Part model, mm, in its own coordinate system. Face numbers are marked on the shaded views. A direction names the side the tool comes from. Coordinates: 2 decimals unless noted, no trailing zeros. Write each loop counter-clockwise with the first axis right and the second up, starting at its lowest first coordinate (ties: lowest second). Pieces come first, ordered by that corner, then holes. Notation, with made-up numbers: (74.25, -32) -> (98.25, -32) arc R18 ccw to (98.25, -27) -> close; hole circle Ø11 at (20, -3.5). An arc over 180 degrees is marked (long way). One line per question, with ' | ' between items. Start each with the question number.
Item 1: Saw through at A-A (y = 0). List the corners of the cut face in (x, z), and give its area (3 significant figures).
Item 2: Pin check, flat tips, straight feed: pin 1 (1.7 mm diameter, centred on y = -2.5, z = 2, fed in from +X); pin 2 (4 mm diameter, centred on y = 1, z = -1, fed in from -X); pin 3 (10 mm diameter, centred on x = -6, y = 3, fed in from +Z); pin 4 (6 mm diameter, centred on x = 5.5, y = -5.5, fed in from -Z). Stop position of each tip, or through.
Item 3: Two-plate mould, pull along Y, no slides. Class the marked faces 1, 2 and 3: pulls with the +Y half, pulls with the -Y half, needs draft (parallel to the pull), parting line crosses it, or undercut.
Item 4: Saw through at B-B (x = -5.5). Count the separate pieces of the cut face and the enclosed holes in it, and give its area (4 significant figures).
Item 5: Probe probe 1 along X at (y, z) = (-3, 3.75); probe 2 along X at (y, z) = (1, -0.75); probe 3 along Y at (x, z) = (-1, 3.5). List the from-to ranges inside material, lowest first. Write a range as [from, to].
Item 6: 3-axis set-ups, long thin cutter, end or side, ignore diameter. For the marked faces 4, 5 and 6: which of +Z, -Z, +X, -X, +Y, -Y reach the whole face in a straight line?
from build123d import *

# Parameters (mm, degrees)
IZIM1_R                          = 14.3
Y_KSEKLIK_EKSTR_ZYON2_DEPTH      = 3
IZIM2_R                          = 13
Y_KSEKLIK_EKSTR_ZYON3_DEPTH      = 1.5
IZIM3_R                          = 13
Y_KSEKLIK_EKSTR_ZYON4_DEPTH      = 1.5
KES_EKSTR_ZYON1_DEPTH            = 7
KES_EKSTR_ZYON3_DEPTH            = 7
IZIM6_R                          = 16
IZIM6_R_2                        = 13
Y_KSEKLIK_EKSTR_ZYON5_DEPTH      = 0.35
Y_KSEKLIK_EKSTR_ZYON5_DEPTH_BACK = 6.65
RADYUS1_R                        = 1
RADYUS2_R                        = 1


with BuildPart() as part:
    # Çizim1 → Yükseklik-Ekstrüzyon2 (new body)
    with BuildSketch(Plane.XY):
        Circle(IZIM1_R)
    extrude(amount=Y_KSEKLIK_EKSTR_ZYON2_DEPTH)

    # Çizim2 → Yükseklik-Ekstrüzyon3 (add)
    with BuildSketch(Plane.XY.offset(3)):
        Circle(IZIM2_R)
    extrude(amount=Y_KSEKLIK_EKSTR_ZYON3_DEPTH)

    # Çizim3 → Yükseklik-Ekstrüzyon4 (add)
    with BuildSketch(Plane(origin=(0, 0, 0), x_dir=(-1, 0, 0), z_dir=(0, 0, -1))):
        Circle(IZIM3_R)
    extrude(amount=Y_KSEKLIK_EKSTR_ZYON4_DEPTH)

    # Çizim4 → Kes-Ekstrüzyon1 (cut)
    with BuildSketch(Plane.XY.offset(4.5)):
        with BuildLine():
            add(Edge.make_bspline(
                [(-0.547346557, 3.558147235), (0.233958313, 12.343828963), (-3.6, 11.184922888)],
                knots=[0, 0, 0, 0.973142828, 0.973142828, 0.973142828], degree=2))
            ThreePointArc((-3.6, 11.184922888), (-3.707741279, 11.149670605), (-3.81513744, 11.113380508))
            ThreePointArc((-3.81513744, 11.113380508), (-10.175798494, 5.875), (-11.532038562, -2.252684312))
            ThreePointArc((-11.532038562, -2.252684312), (-11.509768628, -2.363837165), (-11.48642736, -2.47476999))
            add(Edge.make_bspline(
                [(-3.355119175, -1.305057594), (-10.573090305, -6.374528324), (-11.48642736, -2.47476999)],
                knots=[0, 0, 0, 0.973142828, 0.973142828, 0.973142828], degree=2))
            ThreePointArc((-3.355119175, -1.305057594), (-3.117691454, 1.8), (-0.547346557, 3.558147235))
        make_face()
        with BuildLine():
            add(Edge.make_bspline(
                [(3.355119175, -1.305057594), (10.573090305, -6.374528324), (11.48642736, -2.47476999)],
                knots=[0, 0, 0, 0.973142828, 0.973142828, 0.973142828], degree=2))
            ThreePointArc((11.48642736, -2.47476999), (11.509768628, -2.363837165), (11.532038562, -2.252684312))
            ThreePointArc((11.532038562, -2.252684312), (10.175798494, 5.875), (3.81513744, 11.113380508))
            ThreePointArc((3.81513744, 11.113380508), (3.707741279, 11.149670605), (3.6, 11.184922888))
            add(Edge.make_bspline(
                [(0.547346557, 3.558147235), (-0.233958313, 12.343828963), (3.6, 11.184922888)],
                knots=[0, 0, 0, 0.973142828, 0.973142828, 0.973142828], degree=2))
            ThreePointArc((0.547346557, 3.558147235), (3.117691454, 1.8), (3.355119175, -1.305057594))
        make_face()
        with BuildLine():
            add(Edge.make_bspline(
                [(-2.807772617, -2.253089641), (-10.807048618, -5.969300639), (-7.88642736, -8.710152897)],
                knots=[0, 0, 0, 0.973142828, 0.973142828, 0.973142828], degree=2))
            ThreePointArc((-7.88642736, -8.710152897), (-7.802027349, -8.785833441), (-7.716901122, -8.860696196))
            ThreePointArc((-7.716901122, -8.860696196), (0, -11.75), (7.716901122, -8.860696196))
            ThreePointArc((7.716901122, -8.860696196), (7.802027349, -8.785833441), (7.88642736, -8.710152897))
            add(Edge.make_bspline(
                [(2.807772617, -2.253089641), (10.807048618, -5.969300639), (7.88642736, -8.710152897)],
                knots=[0, 0, 0, 0.973142828, 0.973142828, 0.973142828], degree=2))
            ThreePointArc((2.807772617, -2.253089641), (0, -3.6), (-2.807772617, -2.253089641))
        make_face()
    extrude(amount=-KES_EKSTR_ZYON1_DEPTH, mode=Mode.SUBTRACT)

    # Çizim5 → Kes-Ekstrüzyon3 (cut)
    with BuildSketch(Plane.XY.offset(4.5)):
        with BuildLine():
            Line((-0.243283358, -3.591770205), (-0.243283358, -3.70476627))
            Line((-0.243283358, -3.70476627), (0.246794301, -3.70476627))
            Line((0.246794301, -3.70476627), (0.246794301, -3.591770205))
            Line((0.246794301, -3.591770205), (0.246794301, -1.479558236))
            ThreePointArc((0.246794301, -1.479558236), (1.403567335, -0.529149068), (1.162136883, 0.948386981))
            Line((1.162136883, 0.948386981), (-1.162136883, 0.948386981))
            ThreePointArc((-1.162136883, 0.948386981), (-1.402938645, -0.530813677), (-0.243283358, -1.480139591))
            Line((-0.243283358, -1.480139591), (-0.243283358, -3.591770205))
        make_face()
    extrude(amount=-KES_EKSTR_ZYON3_DEPTH, mode=Mode.SUBTRACT)

    # Çizim6 → Yükseklik-Ekstrüzyon5 (add, two sides)
    with BuildSketch(Plane.XY.offset(4.5)) as y_kseklik_ekstr_zyon5_sk:
        Circle(IZIM6_R)
        Circle(IZIM6_R_2, mode=Mode.SUBTRACT)
    extrude(amount=Y_KSEKLIK_EKSTR_ZYON5_DEPTH)
    extrude(y_kseklik_ekstr_zyon5_sk.sketch, amount=-Y_KSEKLIK_EKSTR_ZYON5_DEPTH_BACK)

    # Radyus1
    radyus1_edges = [part.edges().sort_by_distance(p)[0] for p in [
        (-16, 0, 4.85),
    ]]
    fillet(radyus1_edges, radius=RADYUS1_R)

    # Radyus2
    radyus2_edges = [part.edges().sort_by_distance(p)[0] for p in [
        (-16, 0, -2.15),
    ]]
    fillet(radyus2_edges, radius=RADYUS2_R)


solid = part.part
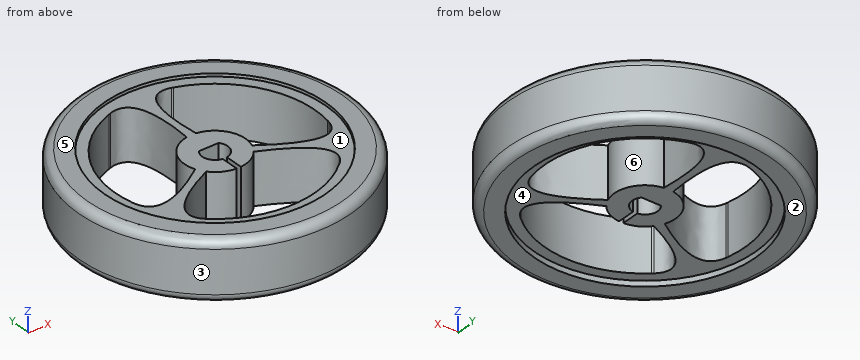
From the geometry:
1) outline: (-16, -1.15) arc R1 ccw to (-15, -2.15) -> (-13, -2.15) -> (-13, -1.5) -> (-11.75, -1.5) -> (-11.75, 4.5) -> (-13, 4.5) -> (-13, 4.85) -> (-15, 4.85) arc R1 ccw to (-16, 3.85) -> close; (-3.6, -1.5) -> (-1.5, -1.5) -> (-1.5, 4.5) -> (-3.6, 4.5) -> close; (1.5, -1.5) -> (3.6, -1.5) -> (3.6, 4.5) -> (1.5, 4.5) -> close; (11.75, -1.5) -> (13, -1.5) -> (13, -2.15) -> (15, -2.15) arc R1 ccw to (16, -1.15) -> (16, 3.85) arc R1 ccw to (15, 4.85) -> (13, 4.85) -> (13, 4.5) -> (11.75, 4.5) -> close | area: 81.3 mm2
2) pin 1: x = 15.91 | pin 2: x = -16 | pin 3: z = 4.5 | pin 4: z = -1.5
3) face 1: undercut | face 2: needs draft | face 3: parting line crosses it
4) separate pieces: 3 | enclosed holes: 0 | area: 67.05 mm2
5) probe 1: [-15.72, -11.32], [-6.04, -4.32], [-1.99, -0.24], [0.25, 1.99], [4.32, 6.04], [11.32, 15.72] | probe 2: [-15.97, -11.71], [-3.46, 3.46], [11.71, 15.97] | probe 3: [-15.97, -11.71], [-3.46, -1.12], [0.95, 3.46], [10.04, 15.97]
6) face 4: -Z | face 5: +Z, +X, -X, +Y, -Y | face 6: +Z, -Z
